Can you work these out from the model? Positions are in its coordinate system, mm. A direction names the side the tool comes from. Round coordinates to 2 decimals unless told otherwise and drop trailing zeros. Loops run counter-clockwise (first coordinate to the right, second up) from the corner with the lowest first, then second, coordinate; pieces in that order, holes last. Notation, with made-up numbers: (9, 83.5) -> (27, 83.5) arc R22 cw to (27, 120.5) -> close; hole circle Ø9 at (-33, 8). An arc over 180 degrees is marked (long way). Answer as a JSON object with one key per item and string values.
```python
from build123d import *

# Parameters (mm, degrees)
F1_DEPTH = 82.55
F3_DEPTH = 190.501


with BuildPart() as f1:
    # F0 (on Front) → F1 (new body)
    with BuildSketch(Plane.XZ):
        Polygon((0, 156.757593), (0, 0), (190.5, 0), (190.5, 12.7), (25.4, 12.7), (25.4, 156.757593), align=None)
    extrude(amount=F1_DEPTH)

    # F2 (on face) → F3 (cut, through all)
    with BuildSketch(Plane(origin=(0, 0, 0), x_dir=(0, -1, 0), z_dir=(-1, 0, 0))):
        with BuildLine():
            ThreePointArc((0, 57.15), (41.275, 98.425), (82.55, 57.15))
            Line((82.55, 57.15), (82.55, 156.757593))
            Line((82.55, 156.757593), (0, 156.757593))
            Line((0, 156.757593), (0, 57.15))
        make_face()
    extrude(amount=-F3_DEPTH, mode=Mode.SUBTRACT)


solid = f1.part
```
Q1. I want a section at D-D, the plane y = -69. Write out the boundary of the cut face in (x, z).
Determined:
{"outline": "(0, 0) -> (190.5, 0) -> (190.5, 12.7) -> (25.4, 12.7) -> (25.4, 87.73) -> (0, 87.73) -> close"}
Q2. On a 3-axis mill with a long thin cutter (end or side, diameter ignored), from which of +Z, -Z, +X, -X, +Y, -Y can I reach the whole of each face in a straight line? I mean faces 1 (the flat face through (25.4, -41, 55)), 2 (the flat face through (94, -41, 0)). Say none if no direction works.
Determined:
{"face 1": "+Z, +X, +Y, -Y", "face 2": "-Z, +X, -X, +Y, -Y"}
Q3. I'm going to push a flat-ended pin straight in: pin 1 (1 mm diameter, centred on y = -43.5, z = 66.5, fed in from +X). Where does the tip first touch, or does it pass through?
Determined:
{"pin 1": "x = 25.4"}
Q4. I want a section at A-A, the plane z = 53.5. Write out the boundary of the cut face in (x, y).
Determined:
{"outline": "(0, -82.55) -> (25.4, -82.55) -> (25.4, 0) -> (0, 0) -> close"}
Q5. I want a section at B-B, the plane x = 148. Write out the boundary of the cut face in (y, z), then the cut area to 3 significant figures.
Determined:
{"outline": "(-82.55, 0) -> (0, 0) -> (0, 12.7) -> (-82.55, 12.7) -> close", "area": "1,050 mm²"}
Q6. I want a section at C-C, the plane y = -34. Write out the boundary of the cut face in (x, z).
Determined:
{"outline": "(0, 0) -> (190.5, 0) -> (190.5, 12.7) -> (25.4, 12.7) -> (25.4, 97.78) -> (0, 97.78) -> close"}
Q7. If I drill on L1, parallel to Z at x = 58, y = -24; L2, parallel to X at y = -44, z = 47.5, over which ranges is the centre line in solid material (lowest first)? Write a range as [from, to].
Determined:
{"L1": "[0, 12.7]", "L2": "[0, 25.4]"}
